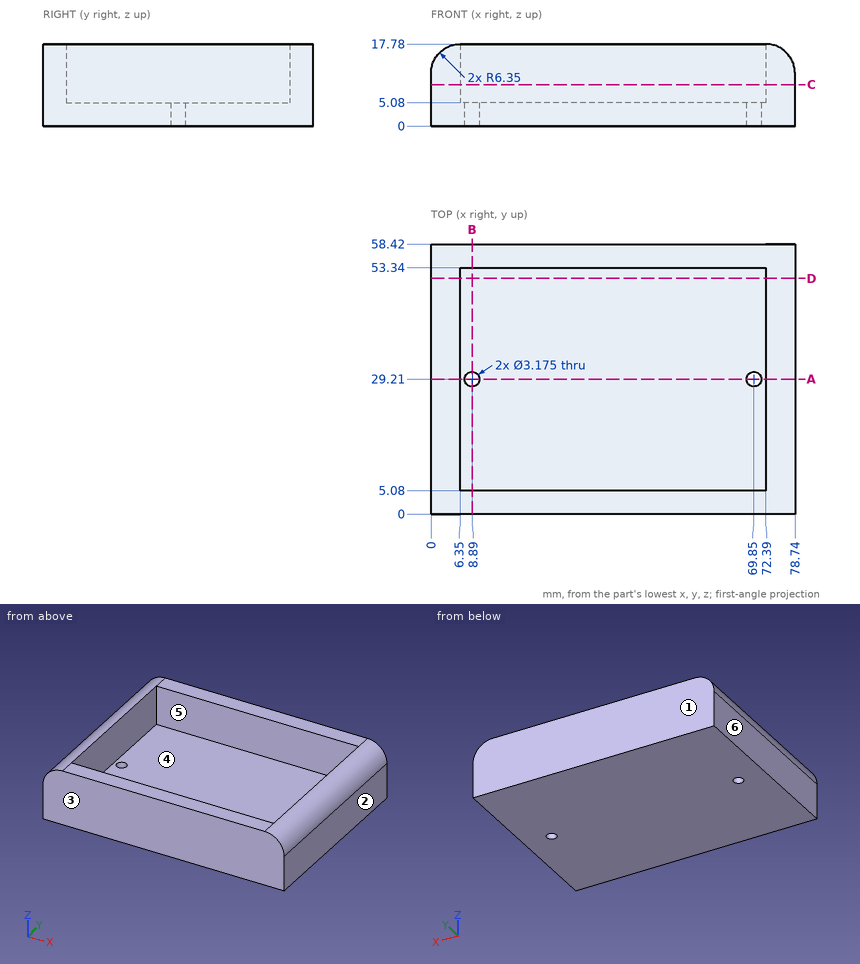
Input: dimensioned drawing with shaded views. Units: mm. Origin: part minimum x, y, z. A direction names the side the tool comes from. Give positions to 0.01 mm unless a question says otherwise; leave off trailing zeros. Loops run counter-clockwise (first coordinate to the right, second up) from the corner with the lowest first, then second, coordinate; pieces in that order, holes last. Notation, with made-up numbers: (-21.5, 8.25) - (33.5, 8.25) arc R20 ccw to (33.5, 23.25) - close; hole circle Ø11 at (51, -22). An arc over 180 degrees is marked (long way). Answer as CSV lines item,"result". Start each with the question number.
(1) Ray query, line 1 along Y through (x, z) = (8.89, 3.3); line 2 along Y through (x, z) = (17, 6.5); line 3 along X through (y, z) = (26, 7.5). Return the intervals inside material, ascending. Write a range as [from, to].
(2) Section query A-A (y = 29.21). Output: boundary loops of the cut face in (x, z), and give its area (3 significant figures).
(3) Section query C-C (z = 9). Output: boundary loops of the cut face in (x, y).
(4) Pin query (flat end, axial travel): P1, Ø3, axis at y = 26, z = 15, coming from the -X side; P2, Ø10, axis at x = 65.5, y = 39, coming from the +Z side. Return the tip coordinate at first contact, or that it passes through.
(5) Section query D-D (y = 51). Output: boundary loops of the cut face in (x, z).
(6) Section query B-B (x = 8.89). Output: boundary loops of the cut face in (y, z).
(7) Reachability of the marked faces 5 and 6 from +Z, -Z, +X, -X, +Y, -Y: full face, straight path, thin tool, end or side. Return the list, or none.
(8) Mould query, pull axis Y, two halves, no side actions, for the marked faces 1, 2, 3 and 4. Classes: +Y half, -Y half, draft (parallel to the pull), parting line (faces both ways), or undercut.
Worked answers:
1,line 1,"y = [0, 27.62], [30.8, 58.42]"
1,line 2,"y = [0, 5.08], [53.34, 58.42]"
1,line 3,"x = [0, 6.35], [72.39, 78.74]"
2,outline,"(0, 0) - (7.3, 0) - (7.3, 5.08) - (6.35, 5.08) - (6.35, 17.78) arc R6.35 ccw to (0, 11.43) - close; (10.48, 0) - (68.26, 0) - (68.26, 5.08) - (10.48, 5.08) - close; (71.44, 0) - (78.74, 0) - (78.74, 11.43) arc R6.35 ccw to (72.39, 17.78) - (72.39, 5.08) - (71.44, 5.08) - close"
2,area,"512 mm^2"
3,outline,"(0, 0) - (78.74, 0) - (78.74, 58.42) - (0, 58.42) - close; hole (6.35, 5.08) - (72.39, 5.08) - (72.39, 53.34) - (6.35, 53.34) - close"
4,P1,"stops at x = 0.35"
4,P2,"stops at z = 5.08"
5,outline,"(0, 0) - (78.74, 0) - (78.74, 11.43) arc R6.35 ccw to (72.39, 17.78) - (72.39, 5.08) - (6.35, 5.08) - (6.35, 17.78) arc R6.35 ccw to (0, 11.43) - close"
6,outline,"(0, 0) - (27.62, 0) - (27.62, 5.08) - (5.08, 5.08) - (5.08, 17.78) - (0, 17.78) - close; (30.8, 0) - (58.42, 0) - (58.42, 17.78) - (53.34, 17.78) - (53.34, 5.08) - (30.8, 5.08) - close"
7,face 5,"+Z"
7,face 6,"+Z, -Z, -X, +Y, -Y"
8,face 1,"+Y half"
8,face 2,"draft"
8,face 3,"-Y half"
8,face 4,"undercut"
